```python
from build123d import *

# Parameters (mm, degrees)
SCALE1_SCALE = 25.4


with BuildPart() as part:
    # Sketch1 → Revolve1 (revolve)
    with BuildSketch(Plane(origin=(0, 0, 0), x_dir=(0, 0, -1), z_dir=(1, 0, 0)), mode=Mode.PRIVATE) as revolve1_sk:
        Polygon((0, 0.725), (24, 0.725), (24, 0.6), (24.18, 0.6), (24.18, 0.725), (24.68, 0.725), (24.68, 0), (0, 0), align=None)
    revolve(revolve1_sk.sketch.rotate(Axis((0, 0, 0), (0, 0, -1)), 90), axis=Axis((0, 0, 0), (0, 0, -1)))


with BuildPart() as part_1:
    # Scale1: scaled about (0, 0, -12.312934608)
    add(part.part.scale(SCALE1_SCALE).moved(Location((0, 0, 300.435604435))))


solid = part_1.part
```
Could you check a few things on this model? Use its own coordinates, in mm. A direction names the side the tool comes from. Coordinates: 2 decimals unless noted, no trailing zeros. Loops run counter-clockwise (first coordinate to the right, second up) from the corner with the lowest first, then second, coordinate; pieces in that order, holes last.
1) Imagine slicing it at A-A (x = 5). List the corners of the cut face in (y, z) for me.
Reported:
outline: (-17.72, -326.44) - (17.72, -326.44) - (17.72, -313.74) - (14.4, -313.74) - (14.4, -309.16) - (17.72, -309.16) - (17.72, 300.44) - (-17.72, 300.44) - (-17.72, -309.16) - (-14.4, -309.16) - (-14.4, -313.74) - (-17.72, -313.74) - close
2) Thinking about a two-plate mould opening in Z: for faces 3 (the face through (0, 0, -326.436)), 4 (the face through (-14.61, 11.21, -320.18)), 5 (the face through (-7, -14, -309.164)), 6 (the face through (0, 0, 300.436)), which applies, released by +Z, released by -Z, zero draft, split by the parting line, or undercut?
Reported:
face 3: released by -Z
face 4: zero draft
face 5: undercut
face 6: released by +Z
3) Please list where these lines run through material, in increasing order: line 1 along Z through (x, y) = (-16, 6); line 2 along X through (y, z) = (2, -159); line 3 along Y through (x, z) = (0, -81) (3 decimals).
Reported:
line 1: z = -326.44 to -313.74, -309.16 to 300.44
line 2: x = -18.31 to 18.31
line 3: y = -18.415 to 18.415
4) Which directions (+Z, -Z, +X, -X, +Y, -Y) give clear straight access to the entire face, cutting with the end or side of a thin tool? Please do faces 1 (the face through (7, -14, -313.736)), 2 (the face through (-14.61, 11.21, -8.63)).
Reported:
face 1: none
face 2: +Z, -Z
5) Imagine slicing it at C-C (y = 7.5). List the corners of the cut face in (x, z) for me.
Reported:
outline: (-16.82, -326.44) - (16.82, -326.44) - (16.82, -313.74) - (13.27, -313.74) - (13.27, -309.16) - (16.82, -309.16) - (16.82, 300.44) - (-16.82, 300.44) - (-16.82, -309.16) - (-13.27, -309.16) - (-13.27, -313.74) - (-16.82, -313.74) - close
6) Will these pins go through, and if not, where does the flat tip stop? pin 1 Ø12 at (x, z) = (4.5, -113.5) entering from -Y (3 decimals); pin 2 Ø6 at (x, z) = (5, -181) entering from -Y; pin 3 Ø6 at (x, z) = (-4.5, 192) entering from +Y.
Reported:
pin 1: stops at y = -18.415
pin 2: stops at y = -18.31
pin 3: stops at y = 18.35
7) Imagine slicing it at B-B (z = -133.5). List the corners of the cut face in (x, y) for me (3 decimals), and give its area (3 significant figures).
Reported:
outline: circle Ø36.83 at (0, 0)
area: 1,070 mm2
